Geometry: final body of the model. Coordinates: model frame, mm. Face numbers are marked on the shaded views. A direction names the side the tool comes from. Coordinates: 2 decimals unless noted, no trailing zeros. Order: outer loops, then holes, each group sorted by start corner. A loop starts at its lowest first (then second) coordinate and runs counter-clockwise, first axis right, second up. Notation, with made-up numbers: M 80.5,-27.75 L 114.5,-27.75 A33 cw 114.5,0.25 Z; hole C 0.25,36 d2. An arc over 180 degrees is marked long. Write item = value, one per line.
from build123d import *

# Parameters (mm, degrees)
F0_W     = 20
F0_H     = 7.5
F1_DEPTH = 35
F3_DEPTH = 15.001
F4_R     = 2.5
F6_DEPTH = 20.001
F5_R     = 2
F7_DEPTH = 6


with BuildPart() as f1:
    # F0 (on Front) → F1 (new body)
    with BuildSketch(Plane.XZ):
        with Locations((-86.824563, -45.478924)):
            Rectangle(F0_W, F0_H)
        Polygon((-76.824563, -41.728924), (-76.824563, -49.228924), (-26.88636, -49.228924), (-25.15431, -48.228924), (-24.818535, -44.838258), (-19.468897, -45.368028), (-15.824563, -43.719141), (-15.824563, -34.228924), (-76.824563, -34.228924), (-76.824563, -39.228924), align=None)
        Polygon((-96.824563, -39.228924), (-96.824563, -41.728924), (-76.824563, -41.728924), (-76.824563, -39.228924), (-76.824563, -34.228924), (-96.824563, -34.228924), align=None)
    extrude(amount=F1_DEPTH)

    # F2 (on face) → F3 (cut, through all)
    with BuildSketch(Plane.XY.offset(-34.228924)):
        Polygon((-76.824563, -30), (-76.824563, -35), (-15.824563, -35), (-15.824563, -25), (-24.818535, -25), (-76.824563, -25), align=None)
        Polygon((-76.824563, 0), (-76.824563, -5), (-76.824563, -10), (-24.818535, -10), (-15.824563, -10), (-15.824563, 0), align=None)
    extrude(amount=-F3_DEPTH, mode=Mode.SUBTRACT)

    # F4 (on face) → F6 (cut, through all)
    with BuildSketch(Plane.YZ.offset(-76.824563)):
        with Locations((-5, -41.728924)):
            Circle(F4_R)
        with Locations((-30, -41.728924)):
            Circle(F4_R)
    extrude(amount=-F6_DEPTH, mode=Mode.SUBTRACT)

    # F5 (on face) → F7 (cut)
    with BuildSketch(Plane(origin=(-96.824563, 0, 0), x_dir=(0, -1, 0), z_dir=(-1, 0, 0))):
        with Locations((22.5, -41.728924)):
            Circle(F5_R)
        with Locations((12.5, -41.728924)):
            Circle(F5_R)
    extrude(amount=-F7_DEPTH, mode=Mode.SUBTRACT)


solid = f1.part
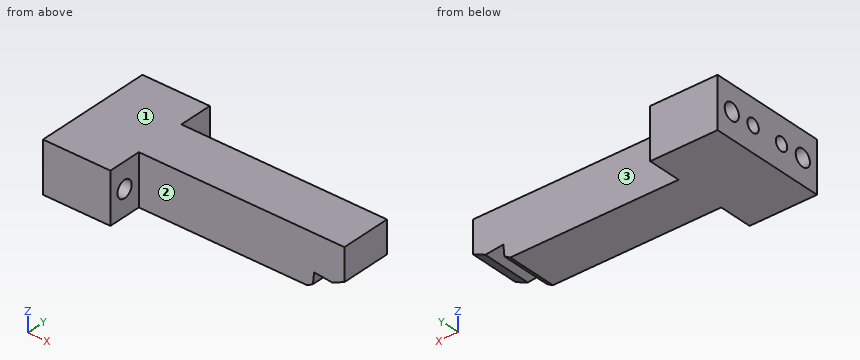
1) Section D-D, the plane z = -38. Return loops of the section in (x, y), and give its area (4 significant figures).
Numbers:
outline = M -96.82,-35 L -76.82,-35 L -76.82,-25 L -15.82,-25 L -15.82,-10 L -76.82,-10 L -76.82,0 L -96.82,0 Z
area = 1,615 mm²
2) Section B-B, the plane z = -42.5. Return loops of the section in (x, y), and give its area (3 significant figures).
Numbers:
outline = M -96.82,-35 L -76.82,-35 L -76.82,-32.38 L -96.82,-32.38 Z; M -96.82,-27.62 L -76.82,-27.62 L -76.82,-25 L -15.82,-25 L -15.82,-10 L -76.82,-10 L -76.82,-7.38 L -96.82,-7.38 L -96.82,-10.65 L -90.82,-10.65 L -90.82,-14.35 L -96.82,-14.35 L -96.82,-20.65 L -90.82,-20.65 L -90.82,-24.35 L -96.82,-24.35 Z; M -96.82,-2.62 L -76.82,-2.62 L -76.82,0 L -96.82,0 Z
area = 1,380 mm²
3) Section C-C, the plane y = -18. Return loops of the section in (x, z), and give its area (3 significant figures).
Numbers:
outline = M -96.82,-49.23 L -26.89,-49.23 L -25.15,-48.23 L -24.82,-44.84 L -19.47,-45.37 L -15.82,-43.72 L -15.82,-34.23 L -96.82,-34.23 Z
area = 1,170 mm²
4) Section A-A, the plane y = -5. Return loops of the section in (x, z).
Numbers:
outline = M -96.82,-49.23 L -76.82,-49.23 L -76.82,-44.23 L -96.82,-44.23 Z; M -96.82,-39.23 L -76.82,-39.23 L -76.82,-34.23 L -96.82,-34.23 Z
5) Set-up query: the marked faces 1, 2 and 3. Return all of +Z, -Z, +X, -X, +Y, -Y with unobstructed straight access to the full face (end or side cutting, diameter ignored); none if empty.
Numbers:
face_1 = +Z, +X, -X, +Y, -Y
face_2 = +Z, -Z, +X, -Y
face_3 = +Z, -Z, +X, +Y
6) Pin query (flat end, axial travel): pin 1 (3 mm diameter, centred on y = -18, z = -44.5, fed in from +X); pin 2 (2 mm diameter, centred on y = -23, z = -42, fed in from -X); pin 3 (4.5 mm diameter, centred on x = -38, z = -44, fed in from +Y); pin 4 (6 mm diameter, centred on y = -5, z = -41.73, fed in from +X). Return the tip coordinate at first contact, or that it passes through.
Numbers:
pin_1 = -15.82
pin_2 = -90.82
pin_3 = -10
pin_4 = -76.82
7) Line query: L1, parallel to Z at x = -93.6, y = -22.5; L2, parallel to X at y = -4.5, z = -38.25; L3, parallel to Y at x = -54.5, z = -35.75. Output: solid intervals per line, ascending.
Numbers:
L1 = -49.23 to -43.73, -39.73 to -34.23
L2 = -96.82 to -76.82
L3 = -25 to -10
